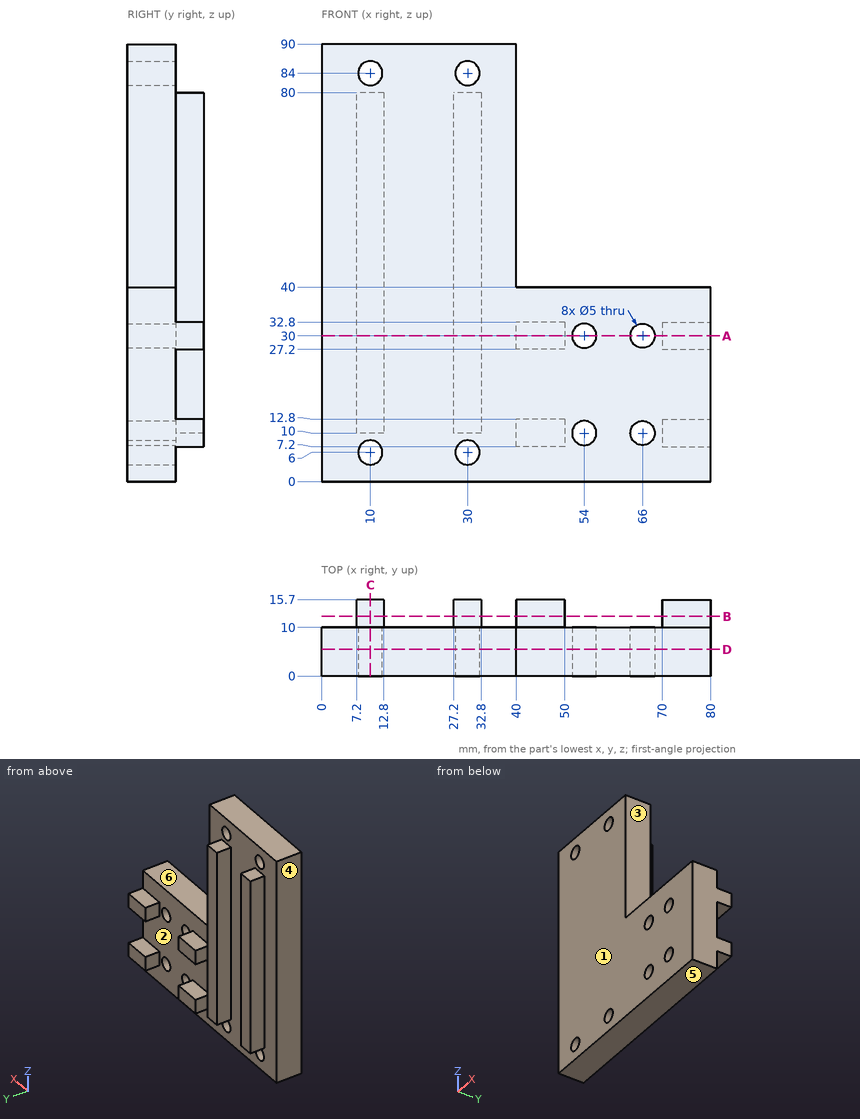
The drawing under review shows one solid part. Ordinate dimensions are in mm from its lowest x, y, z. A direction names the side the tool comes from. Round coordinates to 2 decimals unless told otherwise and drop trailing zeros. Loops run counter-clockwise (first coordinate to the right, second up) from the corner with the lowest first, then second, coordinate; pieces in that order, holes last. Notation, with made-up numbers: (54.25, 39) - (96.25, 39) arc R9 cw to (96.25, 44) - close; hole circle Ø8 at (41.5, 46). An arc over 180 degrees is marked (long way). One line per item, written item: value. Start each with the question number.
1) Consider section B-B on y = 12.25. Give the boundary of the cut face in (x, z).
2) Insertion check: pin 1 Ø3 at (x, y) = (30.5, 14) entering from -Z; pin 2 Ø4.5 at (x, y) = (30, 13.5) entering from +Z; pin 3 Ø4.5 at (x, y) = (45.5, 13) entering from +Z; pin 4 Ø4 at (x, z) = (54, 30) entering from -Y. Each pin has a flat end and moves straight along its axis. Give the tip position at first contact, or say it passes through.
3) Consider section A-A on z = 30. Give the boundary of the cut face in (x, y).
4) Draft analysis for pull direction X (two halves, no side actions). For the marked faces 1, 2, 3 and 4, state which applies: +X half, -X half, draft (parallel to the pull), parting line (faces both ways), or undercut.
5) For the marked faces 5 and 6, list the 3-axis set-ups (+Z, -Z, +X, -X, +Y, -Y) from which the entire face can be reached by the end or side of a thin tool; tool diameter is ignored.
6) To check wall thickness, follow L1, parallel to Z at x = 66, y = 7.5; L2, parallel to X at y = 7.25, z = 6. State the ranges of each line that lie inside material, in increasing order. Write a range as from..to.
7) Consider section D-D on y = 5.5. Give the number of separate pieces and of enclosed holes in the cut face, then the cut area to 3 significant figures.
8) Consider section C-C on x = 10. Give the boundary of the cut face in (y, z).
Reported:
1. outline: (7.2, 10) - (12.8, 10) - (12.8, 80) - (7.2, 80) - close; (27.2, 10) - (32.8, 10) - (32.8, 80) - (27.2, 80) - close; (40, 7.2) - (50, 7.2) - (50, 12.8) - (40, 12.8) - close; (40, 27.2) - (50, 27.2) - (50, 32.8) - (40, 32.8) - close; (70, 7.2) - (80, 7.2) - (80, 12.8) - (70, 12.8) - close; (70, 27.2) - (80, 27.2) - (80, 32.8) - (70, 32.8) - close
2. pin 1: stops at z = 10
2. pin 2: stops at z = 80
2. pin 3: stops at z = 32.8
2. pin 4: passes through
3. outline: (0, 0) - (51.5, 0) - (51.5, 10) - (50, 10) - (50, 15.7) - (40, 15.7) - (40, 10) - (32.8, 10) - (32.8, 15.7) - (27.2, 15.7) - (27.2, 10) - (12.8, 10) - (12.8, 15.7) - (7.2, 15.7) - (7.2, 10) - (0, 10) - close; (56.5, 0) - (63.5, 0) - (63.5, 10) - (56.5, 10) - close; (68.5, 0) - (80, 0) - (80, 15.7) - (70, 15.7) - (70, 10) - (68.5, 10) - close
4. face 1: draft
4. face 2: undercut
4. face 3: +X half
4. face 4: -X half
5. face 5: -Z, +X, -X, +Y, -Y
5. face 6: +Z, +X, +Y, -Y
6. L1: z = 0..7.5, 12.5..27.5, 32.5..40
6. L2: x = 0..7.5, 12.5..27.5, 32.5..80
7. separate pieces: 1
7. enclosed holes: 8
7. area: 5,040 mm^2
8. outline: (0, 0) - (10, 0) - (10, 3.5) - (0, 3.5) - close; (0, 8.5) - (10, 8.5) - (10, 10) - (15.7, 10) - (15.7, 80) - (10, 80) - (10, 81.5) - (0, 81.5) - close; (0, 86.5) - (10, 86.5) - (10, 90) - (0, 90) - close
